Autodesk Inventor part; units mm, degrees
ref_plane "YZ Plane" through (0, 0, 0) normal (1, 0, 0) x (0, 1, 0)
ref_plane "XZ Plane" through (0, 0, 0) normal (0, 1, 0) x (-1, 0, 0)
ref_plane "XY Plane" through (0, 0, 0) normal (0, 0, 1) x (1, 0, 0)
sketch "Sketch1" plane through (0, 0, 0) normal (0, 0, 1) x (1, 0, 0)
  line L0 (0, 0) -> (55.626, 0)
  line L1 (55.626, 0) -> (55.626, -41.275)
  line L2 (55.626, -41.275) -> (0, -41.275)
  line L3 (0, -41.275) -> (0, 0)
  dimension "d0" = 41.275
  dimension "d1" = 55.626
extrude "Extrusion1" add sketch "Sketch1" against normal blind 2.9972
sketch "Sketch2" plane through (0, 0, 0) normal (0, 0, 1) x (1, 0, 0)
  line L0 (0, -41.275) -> (0, 0)
  line L1 (55.626, -41.275) -> (0, -41.275)
  line L2 (20.828, -8.5598) -> (34.798, -8.5598)
  line L3 (34.798, -8.5598) -> (34.798, -17.4498)
  line L4 (34.798, -17.4498) -> (20.828, -17.4498)
  line L5 (20.828, -17.4498) -> (20.828, -8.5598)
  dimension "d4" = 13.97
  dimension "d5" = 8.89
  dimension "d6" = 20.828
  dimension "d7" = 23.8252
extrude "Extrusion2" cut sketch "Sketch2" against normal blind 2.9972
fillet "Fillet1" radius 1.5875 4 edges at (20.828, -17.4498, -1.4986) (20.828, -8.5598, -1.4986) (34.798, -8.5598, -1.4986) (34.798, -17.4498, -1.4986)
sketch "Sketch3" plane through (0, 0, 0) normal (0, 0, 1) x (1, 0, 0)
  line L0 (0, -41.275) -> (0, 0)
  line L1 (55.626, -41.275) -> (0, -41.275)
  line L2 (55.626, 0) -> (55.626, -41.275)
  line L3 (0, -39.6875) -> (55.626, -39.6875)
  line L4 (55.626, -39.6875) -> (55.626, -37.5285)
  line L5 (55.626, -37.5285) -> (0, -37.5285)
  line L6 (0, -37.5285) -> (0, -39.6875)
  dimension "d11" = 1.5875
  dimension "d12" = 2.159
extrude "Extrusion3" cut sketch "Sketch3" against normal blind 1.2446 contours L0 L5 L2 L3
properties part number "Lidar Sensor Case 4 v2 CNC"
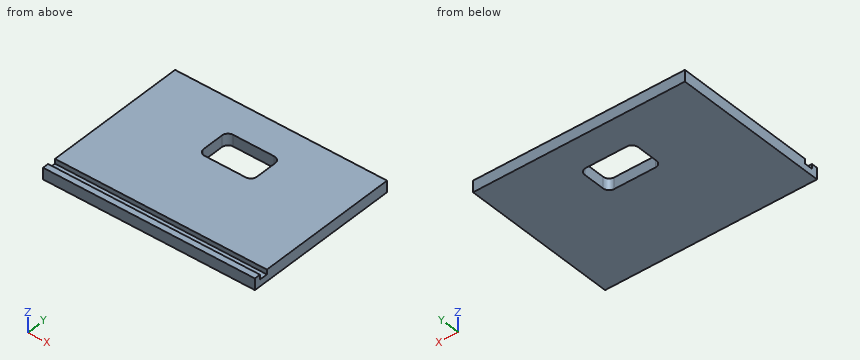
The model under review builds one solid part; all positions refer to its coordinate system, in mm. Round coordinates to 2 decimals unless told otherwise and drop trailing zeros. Order: outer loops, then holes, each group sorted by start corner. A loop starts at its lowest first (then second) coordinate and runs counter-clockwise, first axis right, second up.
Item 1: Add section A-A, the plane x = 32.5. State the section outline as (y, z) points (1 decimal).
Working result:
outline: (-41.3, -3) - (-17.4, -3) - (-17.4, 0) - (-37.5, 0) - (-37.5, -1.2) - (-39.7, -1.2) - (-39.7, 0) - (-41.3, 0) - close; (-8.6, -3) - (0, -3) - (0, 0) - (-8.6, 0) - close
Item 2: Add section C-C, the plane z = -2.2. State the section outline as (x, y) points (1 decimal).
Working result:
outline: (0, -41.3) - (55.6, -41.3) - (55.6, 0) - (0, 0) - close; hole (20.8, -15.9) arc R1.6 ccw to (22.4, -17.4) - (33.2, -17.4) arc R1.6 ccw to (34.8, -15.9) - (34.8, -10.1) arc R1.6 ccw to (33.2, -8.6) - (22.4, -8.6) arc R1.6 ccw to (20.8, -10.1) - close
Item 3: To check wall thickness, follow probe 1 along Y at (x, z) = (32, -0.7) (1 decimal); probe 2 along Y at (x, z) = (20, -0.65) (1 decimal); probe 3 along X at (y, z) = (-10.5, -1.8). State the ranges of each line that lie inside material, in increasing order.
Working result:
probe 1: y = -41.3 to -39.7, -37.5 to -17.4, -8.6 to 0
probe 2: y = -41.3 to -39.7, -37.5 to 0
probe 3: x = 0 to 20.83, 34.8 to 55.63
Item 4: For pin 1 (0.6 mm diameter, centred on x = 15, y = -39, fed in from +Z), flat-tipped, find the tip position at first contact; note if it passes through.
Working result:
pin 1: stops at z = -1.24
Item 5: Add section B-B, the plane y = -13. State the section outline as (x, z) points.
Working result:
outline: (0, -3) - (20.83, -3) - (20.83, 0) - (0, 0) - close; (34.8, -3) - (55.63, -3) - (55.63, 0) - (34.8, 0) - close
Item 6: Add section D-D, the plane x = 9. State the section outline as (y, z) points (1 decimal).
Working result:
outline: (-41.3, -3) - (0, -3) - (0, 0) - (-37.5, 0) - (-37.5, -1.2) - (-39.7, -1.2) - (-39.7, 0) - (-41.3, 0) - close
